from build123d import *

# Parameters (mm, degrees)
F0_W         = 128
F0_H         = 63
F0_W_2       = 125
F0_H_2       = 60
F1_DEPTH     = 31
F0_R         = 4.5
F0_W_3       = 80
F0_H_3       = 58
F0_W_4       = 65
F0_H_4       = 50
F2_DEPTH     = 4
F3_START     = 0.6
F3_DEPTH     = 3.4
F4_R         = 0.3
F6_START     = 10
F6_DEPTH     = 43
F7_W         = 6
F7_H         = 60
F8_DEPTH     = 1
F9_T1_DEPTH  = 29.5
F9_T3_DEPTH  = 33.5
F9_T6_ANGLE  = 90
F9_T8_ANGLE  = 90
F9_T10_ANGLE = 90
F9_T12_ANGLE = 90
F10_SIZE     = 1.5


# Not quite as in the source:
# - a fillet or chamfer that OpenCascade refuses, or shapes differently, is made with other operations: its cross-section is extruded or revolved along the edge and cut away or added


with BuildPart() as f1:
    # F0 (on Front) → F1 (new body)
    with BuildSketch(Plane.XZ):
        Rectangle(F0_W, F0_H)
        Rectangle(F0_W_2, F0_H_2, mode=Mode.SUBTRACT)
    extrude(amount=F1_DEPTH)

    # F0 (on Front) → F2 (join)
    with BuildSketch(Plane.XZ):
        Rectangle(F0_W_2, F0_H_2)
        with Locations((-47.5, -2)):
            Circle(F0_R, mode=Mode.SUBTRACT)
        with Locations((12.5, 0)):
            Rectangle(F0_W_3, F0_H_3, mode=Mode.SUBTRACT)
        with Locations((12.5, 0)):
            Rectangle(F0_W_3, F0_H_3)
        with Locations((15, 0)):
            Rectangle(F0_W_4, F0_H_4, mode=Mode.SUBTRACT)
    extrude(amount=F2_DEPTH)

    # F0 (on Front) → F3 (cut)
    with BuildSketch(Plane.XZ.offset(F3_START)):
        with Locations((12.5, 0)):
            Rectangle(F0_W_3, F0_H_3)
        with Locations((15, 0)):
            Rectangle(F0_W_4, F0_H_4, mode=Mode.SUBTRACT)
    extrude(amount=F3_DEPTH, mode=Mode.SUBTRACT)

    # F4
    f4_edges = [f1.edges().sort_by_distance(p)[0] for p in [
        (64, 0, 0),
        (0, 0, 31.5),
        (-64, 0, 0),
        (0, 0, -31.5),
    ]]
    fillet(f4_edges, radius=F4_R)

    # F5 (on face) → F6 (join)
    with BuildSketch(Plane(origin=(0, 0, 30), x_dir=(1, 0, 0), z_dir=(0, 0, -1)).offset(F6_START)):
        Polygon((-61.5, 19.0501256289), (-62.5, 29), (-62.5, 16.9056187084), align=None)
        Polygon((62.5, 16.9056187084), (62.5, 29), (61.5, 19.0501256289), align=None)
    extrude(amount=F6_DEPTH)

    # F7 (on face) → F8 (join)
    with BuildSketch(Plane.XZ):
        with Locations((-30.5, 0)):
            Rectangle(F7_W, F7_H)
        with Locations((55.5, 0)):
            Rectangle(F7_W, F7_H)
    extrude(amount=F8_DEPTH)

    # F9: fillet of radius 1 on 8 edges, made by hand

    # F9_s2 → F9_t1 (join)
    with BuildSketch(Plane.XZ.offset(1.5)):
        with BuildLine():
            ThreePointArc((62.5, 29), (62.2071067812, 29.7071067812), (61.5, 30))
            Line((61.5, 30), (62.5, 30))
            Line((62.5, 30), (62.5, 29))
        make_face()
        with BuildLine():
            ThreePointArc((-62.5, 29), (-62.2071067812, 29.7071067812), (-61.5, 30))
            Line((-61.5, 30), (-62.5, 30))
            Line((-62.5, 30), (-62.5, 29))
        make_face()
        with BuildLine():
            ThreePointArc((-61.5, -30), (-62.2071067812, -29.7071067812), (-62.5, -29))
            Line((-62.5, -29), (-62.5, -30))
            Line((-62.5, -30), (-61.5, -30))
        make_face()
        with BuildLine():
            ThreePointArc((61.5, -30), (62.2071067812, -29.7071067812), (62.5, -29))
            Line((62.5, -29), (62.5, -30))
            Line((62.5, -30), (61.5, -30))
        make_face()
    extrude(amount=F9_T1_DEPTH)

    # F9_s4 → F9_t3 (cut)
    with BuildSketch(Plane.XZ):
        with BuildLine():
            ThreePointArc((63, 31.5), (63.7071067812, 31.2071067812), (64, 30.5))
            Line((64, 30.5), (64, 31.5))
            Line((64, 31.5), (63, 31.5))
        make_face()
        with BuildLine():
            ThreePointArc((64, -30.5), (63.7071067812, -31.2071067812), (63, -31.5))
            Line((63, -31.5), (64, -31.5))
            Line((64, -31.5), (64, -30.5))
        make_face()
        with BuildLine():
            ThreePointArc((-63, 31.5), (-63.7071067812, 31.2071067812), (-64, 30.5))
            Line((-64, 30.5), (-64, 31.5))
            Line((-64, 31.5), (-63, 31.5))
        make_face()
        with BuildLine():
            ThreePointArc((-64, -30.5), (-63.7071067812, -31.2071067812), (-63, -31.5))
            Line((-63, -31.5), (-64, -31.5))
            Line((-64, -31.5), (-64, -30.5))
        make_face()
    extrude(amount=F9_T3_DEPTH, mode=Mode.SUBTRACT)

    # F9_s5 → F9_t6 (revolve, cut)
    with BuildSketch(Plane.YZ.offset(-63)):
        with BuildLine():
            ThreePointArc((0, -31.2), (-0.0878679656, -31.4121320344), (-0.3, -31.5))
            Line((-0.3, -31.5), (0, -31.5))
            Line((0, -31.5), (0, -31.2))
        make_face()
    revolve(axis=Axis((-63, 0, -30.5), (0, 1, 0)), revolution_arc=F9_T6_ANGLE, mode=Mode.SUBTRACT)

    # F9_s7 → F9_t8 (revolve, cut)
    with BuildSketch(Plane.XY.offset(30.5)):
        with BuildLine():
            ThreePointArc((-63.7, 0), (-63.9121320344, -0.0878679656), (-64, -0.3))
            Line((-64, -0.3), (-64, 0))
            Line((-64, 0), (-63.7, 0))
        make_face()
    revolve(axis=Axis((-63, 0, 30.5), (0, 1, 0)), revolution_arc=F9_T8_ANGLE, mode=Mode.SUBTRACT)

    # F9_s9 → F9_t10 (revolve, cut)
    with BuildSketch(Plane.XY.offset(-30.5)):
        with BuildLine():
            ThreePointArc((63.7, 0), (63.9121320344, -0.0878679656), (64, -0.3))
            Line((64, -0.3), (64, 0))
            Line((64, 0), (63.7, 0))
        make_face()
    revolve(axis=Axis((63, 0, -30.5), (0, 1, 0)), revolution_arc=F9_T10_ANGLE, mode=Mode.SUBTRACT)

    # F9_s11 → F9_t12 (revolve, cut)
    with BuildSketch(Plane.YZ.offset(63)):
        with BuildLine():
            ThreePointArc((0, 31.2), (-0.0878679656, 31.4121320344), (-0.3, 31.5))
            Line((-0.3, 31.5), (0, 31.5))
            Line((0, 31.5), (0, 31.2))
        make_face()
    revolve(axis=Axis((63, 0, 30.5), (0, 1, 0)), revolution_arc=F9_T12_ANGLE, mode=Mode.SUBTRACT)

    # F10
    f10_edges = [f1.edges().sort_by_distance(p)[0] for p in [
        (-52, -4, -2),
    ]]
    chamfer(f10_edges, length=F10_SIZE)


solid = f1.part
Geometry check sheet. Reference: the model listing, model coordinates, mm. A direction names the side the tool comes from. Coordinates: 2 decimals unless noted, no trailing zeros. Order: outer loops, then holes, each group sorted by start corner. A loop starts at its lowest first (then second) coordinate and runs counter-clockwise, first axis right, second up. Notation, with made-up numbers: (-9, 88.5) -> (34, 88.5) arc R23 ccw to (34, 111.5) -> close; hole circle Ø8 at (33.5, 59.5). An arc over 180 degrees is marked (long way). Use a Markdown table: item, result. Add a question column.
1. Material ranges on L1, parallel to Z at x = 43, y = -23.5; L2, parallel to X at y = -20.5, z = 27; L3, parallel to Z at x = -47, y = -1, recorded low to high.
2. Set-up check for faces 5 (the face through (-1, -15, -31.5)), 6 (the face through (52.5, -2, 0)), 7 (the face through (-62.5, -14, 0)): record each of +Z, -Z, +X, -X, +Y, -Y from which the full face is reachable in a straight line by a thin tool's end or side.
3. Go/stop test with flat-tipped pins: pin 1 Ø18 at (x, z) = (-13.5, -11.5) entering from -Y; pin 2 Ø0.7 at (y, z) = (0, 0) entering from -X. Record where each tip stops, or that it passes through.
4. Cross-section at A-A (z = -10.5). Enter the section's corners in (x, y).
5. Cross-section at D-D (z = -2). Give the number of separate pieces and of enclosed holes in the cut face, and give its area (3 significant figures).
6. Cross-section at B-B (x = 32). Enter the section's corners in (y, z).
7. Cross-section at C-C (y = -11). Enter the section's corners in (x, z), and give its area (3 significant figures).
8. Mould release check, pull along X, two halves, no side actions. Record for faces 1 (the face through (-29, 0, 0)), 2 (the face through (64, -15, 0)), 3 (the face through (-1, -17, 30)), 4 (the face through (-64, -15, 0)): pulls with the +X half, pulls with the -X half, needs draft (parallel to the pull), parting line crosses it, or undercut.
Filled sheet:
| question | item | result |
|---|---|---|
| 1 | L1 | -31.5 to -30, 30 to 31.5 |
| 1 | L2 | -64 to -62.5, 62.5 to 64 |
| 1 | L3 | -31.5 to -6.47, 2.47 to 31.5 |
| 2 | face 5 | -Z, +X, -X, +Y, -Y |
| 2 | face 6 | -Y |
| 2 | face 7 | none |
| 3 | pin 1 | y = -0.6 |
| 3 | pin 2 | x = -64 |
| 4 | outline | (-64, -31) -> (-62.5, -31) -> (-62.5, -29) -> (-61.5, -19.05) -> (-62.5, -16.91) -> (-62.5, -4) -> (-27.5, -4) -> (-27.5, -0.6) -> (-17.5, -0.6) -> (-17.5, 0) -> (-63.7, 0) arc R0.3 ccw to (-64, -0.3) -> close; (47.5, -0.6) -> (52.5, -0.6) -> (52.5, -4) -> (62.5, -4) -> (62.5, -16.91) -> (61.5, -19.05) -> (62.5, -29) -> (62.5, -31) -> (64, -31) -> (64, -0.3) arc R0.3 ccw to (63.7, 0) -> (47.5, 0) -> close |
| 5 | separate pieces | 3 |
| 5 | enclosed holes | 0 |
| 5 | area | 256 mm2 |
| 6 | outline | (-31, -31.5) -> (-0.3, -31.5) arc R0.3 ccw to (0, -31.2) -> (0, -25) -> (-0.6, -25) -> (-0.6, -29) -> (-4, -29) -> (-4, -30) -> (-31, -30) -> close; (-31, 30) -> (-4, 30) -> (-4, 29) -> (-0.6, 29) -> (-0.6, 25) -> (0, 25) -> (0, 31.2) arc R0.3 ccw to (-0.3, 31.5) -> (-31, 31.5) -> close |
| 7 | outline | (-64, -30.5) arc R1 ccw to (-63, -31.5) -> (63, -31.5) arc R1 ccw to (64, -30.5) -> (64, 30.5) arc R1 ccw to (63, 31.5) -> (-63, 31.5) arc R1 ccw to (-64, 30.5) -> close; hole (-62.5, -29) arc R1 ccw to (-61.5, -30) -> (61.5, -30) arc R1 ccw to (62.5, -29) -> (62.5, 29) arc R1 ccw to (61.5, 30) -> (-61.5, 30) arc R1 ccw to (-62.5, 29) -> close |
| 7 | area | 564 mm2 |
| 8 | face 1 | needs draft |
| 8 | face 2 | pulls with the +X half |
| 8 | face 3 | undercut |
| 8 | face 4 | pulls with the -X half |
